Job drawing, mm, ordinate dimensions from the low corner. One solid piece. Give positions to 0.01 mm unless a question says otherwise; leave off trailing zeros. Order: outer loops, then holes, each group sorted by start corner. A loop starts at its lowest first (then second) coordinate and runs counter-clockwise, first axis right, second up. Notation, with made-up numbers: M -35,-31 L -2,-31 A28 ccw -2,7 Z; hole C -33.75,65 d1. An arc over 180 degrees is marked long. One line per question, with ' | ' between items.
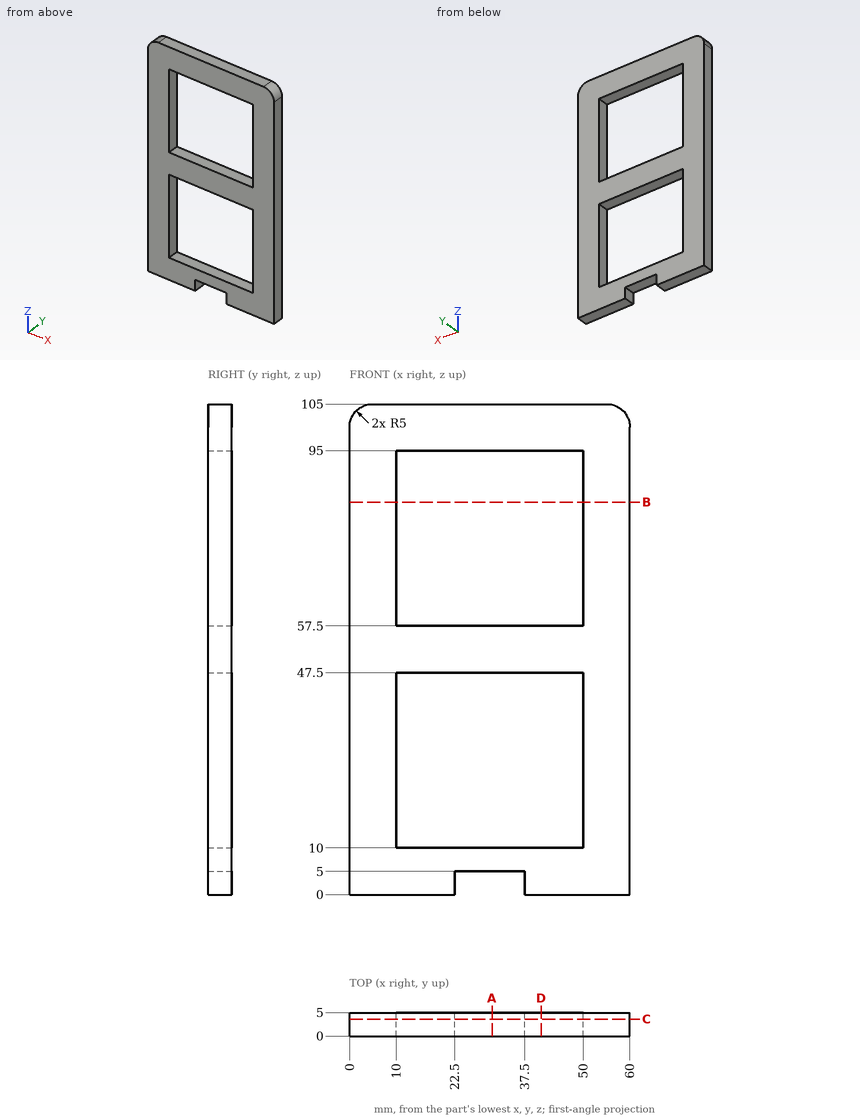
1. Slice it at C-C on y = 3.6. Give the cut face in (x, z).
Worked out:
outline: M 0,0 L 22.5,0 L 22.5,5 L 37.5,5 L 37.5,0 L 60,0 L 60,100 A5 ccw 55,105 L 5,105 A5 ccw 0,100 Z; hole M 10,10 L 50,10 L 50,47.5 L 10,47.5 Z; hole M 10,57.5 L 50,57.5 L 50,95 L 10,95 Z
2. Probe L1, parallel to Z at x = 44, y = 1.7; L2, parallel to Z at x = 34, y = 1.5; L3, parallel to X at y = 3.05, z = 12.5. List the from-to ranges inside material, lowest first. Write a range as from..to.
Worked out:
L1: z = 0..10, 47.5..57.5, 95..105 | L2: z = 5..10, 47.5..57.5, 95..105 | L3: x = 0..10, 50..60
3. Slice it at D-D on x = 41. Give the cut face in (y, z), then the cut area to 3 significant figures.
Worked out:
outline: M 0,0 L 5,0 L 5,10 L 0,10 Z; M 0,47.5 L 5,47.5 L 5,57.5 L 0,57.5 Z; M 0,95 L 5,95 L 5,105 L 0,105 Z | area: 150 mm2
4. Drop a flat-ended pin along its axis: pin 1 (2.5 mm diameter, centred on x = 29, y = 2.5, fed in from -Z). Give the stop position or say it passes through.
Worked out:
pin 1: stops at z = 5
5. Slice it at B-B on z = 84. Give the cut face in (x, y).
Worked out:
outline: M 0,0 L 10,0 L 10,5 L 0,5 Z; M 50,0 L 60,0 L 60,5 L 50,5 Z
6. Slice it at A-A on x = 30.5. Give the cut face in (y, z), then the cut area to 3 significant figures.
Worked out:
outline: M 0,5 L 5,5 L 5,10 L 0,10 Z; M 0,47.5 L 5,47.5 L 5,57.5 L 0,57.5 Z; M 0,95 L 5,95 L 5,105 L 0,105 Z | area: 125 mm2
